Read the model definition and answer for the solid it produces. Units are mm, in the model's axes. A direction names the side the tool comes from. Give positions to 0.01 mm unless a question says otherwise; leave off trailing zeros. Loops run counter-clockwise (first coordinate to the right, second up) from the corner with the lowest first, then second, coordinate; pieces in that order, holes last. Notation, with made-up numbers: (-4.5, 19) -> (32.5, 19) arc R13 cw to (32.5, 37) -> close; hole circle Ø1 at (12, 58.25). An arc over 180 degrees is marked (long way). Write each question's results on one line, items separated by ' | '. Start each with the question number.
Item 1: Each of these flat-tipped pins is pushed along its axis until it touches: P1, Ø5, axis at x = -50.5, z = 51, coming from the -Y side; P2, Ø1.5, axis at x = -29, y = -32, coming from the +Z side; P3, Ø1.5, axis at x = -31, y = 8, coming from the -Z side; P4, Ø4, axis at y = 2.5, z = 22, coming from the +X side. Where does it stop, or does it pass through?
Item 2: Section B-B on y = -19 is taken. Write down the section's boundary in (x, z), and give its area (3 significant figures).
Item 3: Determine the mould class of faces 4 (the flat face through (-1, 1, 101.6)), 5 (the cylindrical face through (-30.235, 23.183, 38.311)), 6 (the cylindrical face through (-45.497, 2.002, 31.483)) for opening direction X: +X half, -X half, draft (parallel to the pull), parting line (faces both ways), or undercut.
Item 4: Section A-A on x = 0 is taken. Write down the section's boundary in (y, z).
Item 5: Find the intervals of material crossed by line 1 (Y direction, x = 0, z = 16.5); line 2 (Y direction, x = 0, z = 60), in increasing order.
Item 6: Section D-D on z = 87.5 is taken. Write down the section's boundary in (x, y).
Item 7: Which of the six approach directions +Z, -Z, +X, -X, +Y, -Y give full straight-line access (tool end or side, diameter ignored) to faces 1 (the flat face through (-1, -1, 77.709)), 2 (the cylindrical face through (62.018, 19.53, 6.261)), 3 (the cylindrical face through (38.318, 12.067, 75.844))?
Item 8: Section C-C on z = 21.5 is taken. Write down the section's boundary in (x, y).
```python
from build123d import *

# Parameters (mm, degrees)
F0_R     = 65.020167
F1_DEPTH = 12.7
F2_R     = 45.541471
F3_DEPTH = 38.1
F4_R     = 40.172853
F5_DEPTH = 50.8
F6_R     = 38.1
F7_DEPTH = 77.709325


with BuildPart() as f1:
    # F0 (on Top) → F1 (new body)
    with BuildSketch(Plane.XY):
        Circle(F0_R)
    extrude(amount=F1_DEPTH)

    # F2 (on face) → F3 (join)
    with BuildSketch(Plane.XY.offset(12.7)):
        Circle(F2_R)
    extrude(amount=F3_DEPTH)

    # F4 (on face) → F5 (join)
    with BuildSketch(Plane.XY.offset(50.8)):
        Circle(F4_R)
    extrude(amount=F5_DEPTH)

    # F6 (on face) → F7 (cut)
    with BuildSketch(Plane(origin=(0, 0, 0), x_dir=(1, 0, 0), z_dir=(0, 0, -1))):
        Circle(F6_R)
    extrude(amount=-F7_DEPTH, mode=Mode.SUBTRACT)


solid = f1.part
```
Findings:
1) P1: through | P2: z = 50.8 | P3: z = 77.71 | P4: x = 45.54
2) outline: (-62.18, 0) -> (-33.02, 0) -> (-33.02, 77.71) -> (33.02, 77.71) -> (33.02, 0) -> (62.18, 0) -> (62.18, 12.7) -> (41.39, 12.7) -> (41.39, 50.8) -> (35.4, 50.8) -> (35.4, 101.6) -> (-35.4, 101.6) -> (-35.4, 50.8) -> (-41.39, 50.8) -> (-41.39, 12.7) -> (-62.18, 12.7) -> close | area: 3,200 mm2
3) face 4: draft | face 5: undercut | face 6: parting line
4) outline: (-65.02, 0) -> (-38.1, 0) -> (-38.1, 77.71) -> (38.1, 77.71) -> (38.1, 0) -> (65.02, 0) -> (65.02, 12.7) -> (45.54, 12.7) -> (45.54, 50.8) -> (40.17, 50.8) -> (40.17, 101.6) -> (-40.17, 101.6) -> (-40.17, 50.8) -> (-45.54, 50.8) -> (-45.54, 12.7) -> (-65.02, 12.7) -> close
5) line 1: -45.54 to -38.1, 38.1 to 45.54 | line 2: -40.17 to -38.1, 38.1 to 40.17
6) outline: circle Ø80.35 at (0, 0)
7) face 1: -Z | face 2: +Z, -Z | face 3: +Z
8) outline: circle Ø91.08 at (0, 0); hole circle Ø76.2 at (0, 0)
